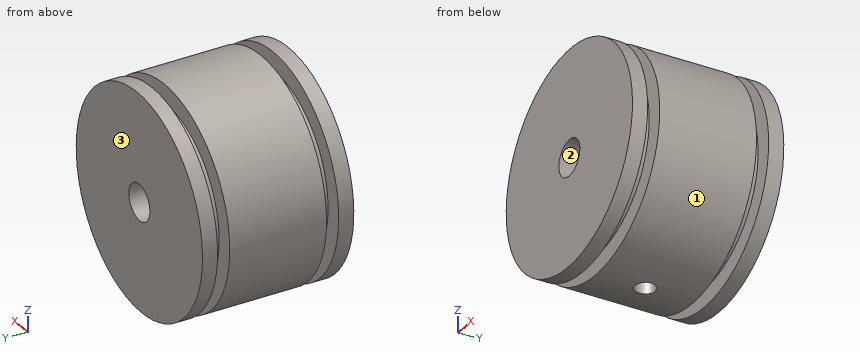
```python
from build123d import *

# Parameters (mm, degrees)
SKETCH2_R          = 1.65
CUT_EXTRUDE1_DEPTH = 36.67912555


with BuildPart() as part:
    # Sketch1 → Revolve1 (revolve)
    with BuildSketch(Plane.XY, mode=Mode.PRIVATE) as revolve1_sk:
        Polygon((10, 0), (18, 0), (18, 2.5), (15, 2.5), (15, 4.5), (18, 4.5), (18, 20.5), (15, 20.5), (15, 22.5), (18, 22.5), (18, 25), (3, 25), (3, 0), align=None)
    revolve(revolve1_sk.sketch.rotate(Axis((0, 0, 0), (0, 1, 0)), 90), axis=Axis((0, 0, 0), (0, 1, 0)))

    # Sketch2 → Cut-Extrude1 (cut, through all)
    with BuildSketch(Plane.XY):
        with Locations(Location((0, 12.5, 0), (0, 0, 90))):
            Circle(SKETCH2_R)
    extrude(amount=-CUT_EXTRUDE1_DEPTH, mode=Mode.SUBTRACT)


solid = part.part
```
The listing builds one solid part. Answer for the finished solid, in the listing's coordinates (mm). Face numbers are marked on the shaded views. Coordinates: 2 decimals unless noted, no trailing zeros. Loops run counter-clockwise (first coordinate to the right, second up) from the corner with the lowest first, then second, coordinate; pieces in that order, holes last. Notation, with made-up numbers: (72, 51.25) - (86, 51.25) arc R23 ccw to (86, 77.25) - close; hole circle Ø8 at (33.5, -31.5). An arc over 180 degrees is marked (long way). Write item = value, one per line.
1) Each of these flat-tipped pins is pushed along its axis until it touches: P1, Ø6, axis at y = 12.5, z = 0, coming from the -X side; P2, Ø3.5, axis at x = 0, z = 0, coming from the -Y side; P3, Ø8, axis at y = 3.5, z = -11.5, coming from the -X side; P4, Ø6, axis at x = -10.5, y = 4.5, coming from the +Z side. Where does it stop, or does it pass through?
Responses:
P1 = -18
P2 = through
P3 = -16.3
P4 = 16.36
2) Section A-A (x = 0) is taken. Determine the outline of the cut face in (y, z), plus the area to 4 significant figures.
Responses:
outline = (0, -18) - (2.5, -18) - (2.5, -15) - (4.5, -15) - (4.5, -18) - (10.85, -18) - (10.85, -3) - (0, -3) - close; (0, 3) - (25, 3) - (25, 18) - (22.5, 18) - (22.5, 15) - (20.5, 15) - (20.5, 18) - (4.5, 18) - (4.5, 15) - (2.5, 15) - (2.5, 18) - (0, 18) - close; (14.15, -18) - (20.5, -18) - (20.5, -15) - (22.5, -15) - (22.5, -18) - (25, -18) - (25, -3) - (14.15, -3) - close
area = 676.5 mm^2
3) Section B-B (z = 0) is taken. Determine the outline of the cut face in (x, y), plus the area to 3 significant figures.
Responses:
outline = (-18, 0) - (-3, 0) - (-3, 25) - (-18, 25) - (-18, 22.5) - (-15, 22.5) - (-15, 20.5) - (-18, 20.5) - (-18, 4.5) - (-15, 4.5) - (-15, 2.5) - (-18, 2.5) - close; (3, 0) - (18, 0) - (18, 2.5) - (15, 2.5) - (15, 4.5) - (18, 4.5) - (18, 20.5) - (15, 20.5) - (15, 22.5) - (18, 22.5) - (18, 25) - (3, 25) - close
area = 726 mm^2
4) Section C-C (z = -7) is taken. Determine the outline of the cut face in (x, y).
Responses:
outline = (-16.58, 0) - (16.58, 0) - (16.58, 2.5) - (13.27, 2.5) - (13.27, 4.5) - (16.58, 4.5) - (16.58, 20.5) - (13.27, 20.5) - (13.27, 22.5) - (16.58, 22.5) - (16.58, 25) - (-16.58, 25) - (-16.58, 22.5) - (-13.27, 22.5) - (-13.27, 20.5) - (-16.58, 20.5) - (-16.58, 4.5) - (-13.27, 4.5) - (-13.27, 2.5) - (-16.58, 2.5) - close; hole circle Ø3.3 at (0, 12.5)
5) Section D-D (x = 15.5) is taken. Determine the outline of the cut face in (y, z).
Responses:
outline = (0, -9.15) - (2.5, -9.15) - (2.5, 9.15) - (0, 9.15) - close; (4.5, -9.15) - (20.5, -9.15) - (20.5, 9.15) - (4.5, 9.15) - close; (22.5, -9.15) - (25, -9.15) - (25, 9.15) - (22.5, 9.15) - close
6) Find the intervals of material crossed by line 1 along Y through (x, z) = (6.5, 15.5); line 2 along X through (y, z) = (5.75, 0); line 3 along X through (y, z) = (23, -2.5), in increasing order.
Responses:
line_1 = 0 to 2.5, 4.5 to 20.5, 22.5 to 25
line_2 = -18 to -3, 3 to 18
line_3 = -17.83 to -1.66, 1.66 to 17.83
7) Determine the mould class of the marked faces 1, 2 and 3 for opening direction Z: pulls with the +Z half, pulls with the -Z half, needs draft (parallel to the pull), parting line crosses it, or undercut.
Responses:
face_1 = parting line crosses it
face_2 = undercut
face_3 = needs draft
